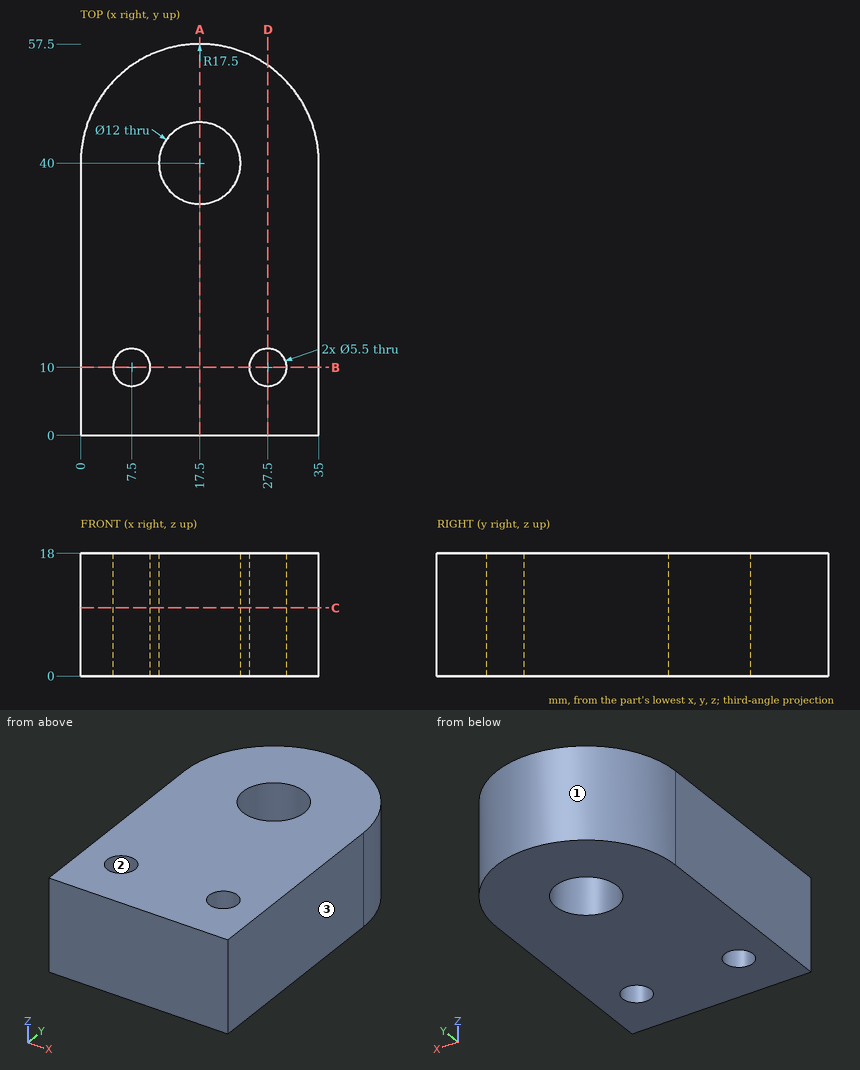
Could you check a few things on this drawing? It's one solid part, dimensions in mm from its lowest x, y, z. Coordinates: 2 decimals unless noted, no trailing zeros. Write each loop counter-clockwise with the first axis right and the second up, starting at its lowest first coordinate (ties: lowest second). Pieces come first, ordered by that corner, then holes. Notation, with made-up numbers: M 79,-15 L 133,-15 A20 cw 133,7 Z; hole C 31.25,-31.5 d3. An arc over 180 degrees is marked long. Answer as CSV lines item,"result". Start each with the question number.
Q1. Will these pins go through, and if not, where does the flat tip stop? pin 1 Ø6 at (x, y) = (8.5, 30.5) entering from -Z; pin 2 Ø1.5 at (x, z) = (20, 11) entering from +Y; pin 3 Ø3 at (y, z) = (48, 10.5) entering from -X; pin 4 Ø9.5 at (x, y) = (17.5, 40) entering from -Z.
Q2. Suppose I cut it at A-A, the plane x = 17.5. List the corners of the cut face in (y, z) for me, then the cut area to 3 significant figures.
Q3. Suppose I cut it at D-D, the plane x = 27.5. List the corners of the cut face in (y, z) for me.
Q4. If we mould it in two halves opening along Y, with no side actions, what happens to the marked faces 1, 2 and 3? For each: pulls with the +Y half, pulls with the -Y half, needs draft (parallel to the pull), parting line crosses it, or undercut.
Q5. Suppose I cut it at C-C, the plane z = 10. List the corners of the cut face in (x, y) for me.
Q6. I need wall thicknesses on probe 1 along Y at (x, z) = (17.5, 11.25); probe 2 along Y at (x, z) = (7.5, 11); probe 3 along X at (y, z) = (8.5, 12.5). Which ranges of each line are inside material? Lowest first, please. Write a range as [from, to].
Q7. Suppose I cut it at B-B, the plane y = 10. List the corners of the cut face in (x, z) for me.
Entries:
1,pin 1,"stops at z = 0"
1,pin 2,"stops at y = 57.41"
1,pin 3,"stops at x = 1.25"
1,pin 4,"passes through"
2,outline,"M 0,0 L 34,0 L 34,18 L 0,18 Z; M 46,0 L 57.5,0 L 57.5,18 L 46,18 Z"
2,area,"819 mm²"
3,outline,"M 0,0 L 7.25,0 L 7.25,18 L 0,18 Z; M 12.75,0 L 54.36,0 L 54.36,18 L 12.75,18 Z"
4,face 1,"pulls with the +Y half"
4,face 2,"undercut"
4,face 3,"needs draft"
5,outline,"M 0,0 L 35,0 L 35,40 A17.5 ccw 0,40 Z; hole C 7.5,10 d5.5; hole C 17.5,40 d12; hole C 27.5,10 d5.5"
6,probe 1,"y = [0, 34], [46, 57.5]"
6,probe 2,"y = [0, 7.25], [12.75, 54.36]"
6,probe 3,"x = [0, 5.2], [9.8, 25.2], [29.8, 35]"
7,outline,"M 0,0 L 4.75,0 L 4.75,18 L 0,18 Z; M 10.25,0 L 24.75,0 L 24.75,18 L 10.25,18 Z; M 30.25,0 L 35,0 L 35,18 L 30.25,18 Z"
